```python
from build123d import *

# Parameters (mm, degrees)
SKETCH1_R           = 6
BOSS_EXTRUDE1_DEPTH = 5


with BuildPart() as part:
    # Sketch1 → Boss-Extrude1 (new, symmetric)
    with BuildSketch(Plane.XY):
        with BuildLine():
            ThreePointArc((0, -10), (9.930121511, -1.180121511), (2.34375, 9.721462644))
            Line((2.34375, 9.721462644), (-58.140625, 24.30365661))
            ThreePointArc((-58.140625, 24.30365661), (-86.874486916, 10.08750952), (-77.994140625, -20.716274476))
            ThreePointArc((-77.994140625, -20.716274476), (-72.385268542, -20.708675871), (-70.3125, -15.496849478))
            ThreePointArc((-70.3125, -15.496849478), (-71.576881743, -7.794228634), (-72, 0))
            ThreePointArc((-72, 0), (-64, 8), (-56, 0))
            ThreePointArc((-56, 0), (-55.051774585, -10.261681883), (-52.239210176, -20.175849925))
            ThreePointArc((-52.239210176, -20.175849925), (-46.886715458, -25.748635939), (-39.160382636, -25.843107024))
            Line((-39.160382636, -25.843107024), (0, -10))
        make_face()
        Circle(SKETCH1_R, mode=Mode.SUBTRACT)
    extrude(amount=BOSS_EXTRUDE1_DEPTH, both=True)


solid = part.part
```
Can you work these out from the model? Positions are in its coordinate system, mm. A direction names the side the tool comes from. Coordinates: 2 decimals unless noted, no trailing zeros. Loops run counter-clockwise (first coordinate to the right, second up) from the corner with the lowest first, then second, coordinate; pieces in that order, holes last.
1) Imagine slicing it at D-D on y = 5. List the corners of the cut face in (x, z) for me (3 decimals).
2) I need wall thicknesses on probe 1 along X at (y, z) = (-0.5, 2.25) (1 decimal); probe 2 along Y at (x, z) = (0, 2.25); probe 3 along X at (y, z) = (-14.5, 0). Which ranges of each line are inside material? Lowest first, please.
3) Imagine slicing it at A-A on z = 1. List the corners of the cut face in (x, y) for me, plus the area to 3 significant figures.
4) Imagine slicing it at C-C on x = -64. List the corners of the cut face in (y, z) for me.
5) For pin 1 (11 mm diameter, centred on x = 0, y = 0, fed in from +Z); pin 2 (1.5 mm diameter, centred on x = -67, z = 0, fed in from +Y); pin 3 (1.5 mm diameter, centred on x = -24, z = -1, fed in from -Y); pin 4 (4 mm diameter, centred on y = 10, z = 2.5, fed in from -X), each with a flat end and sliding along its axis, tell me the tip position at first contact or that it passes through.
6) Which directions (+Z, -Z, +X, -X, +Y, -Y) give clear straight access to the entire face, cutting with the end or side of a thin tool? Please do faces 5 (the flat face through (-19.85, -18.03, 0.07)), 6 (the cylindrical face through (-71.565, -7.903, 0.07)).
7) Imagine slicing it at B-B on y = -2. List the corners of the cut face in (x, z) for me.
8) Thinking about a two-plate mould opening in Y: for faces 1 (the cylindrical face through (-64, 8, 0)), 2 (the flat face through (-40, 0, 5)), 3 (the cylindrical face through (9.9, -1.4, 0.1)), 4 (the cylindrical face through (-55.08, -10.12, 0.07)), which applies, pulls with the +Y half, pulls with the -Y half, needs draft (parallel to the pull), parting line crosses it, or undercut?
Completed:
1. outline: (-88.495, -5) - (-70.245, -5) - (-70.245, 5) - (-88.495, 5) - close; (-57.755, -5) - (-3.317, -5) - (-3.317, 5) - (-57.755, 5) - close; (3.317, -5) - (8.66, -5) - (8.66, 5) - (3.317, 5) - close
2. probe 1: x = -89 to -72, -56 to -6, 6 to 10
2. probe 2: y = -10 to -6, 6 to 10.29
2. probe 3: x = -84.37 to -70.52, -54.09 to -11.12
3. outline: (-77.99, -20.72) arc R5 ccw to (-70.31, -15.5) arc R72 cw to (-72, 0) arc R8 cw to (-56, 0) arc R56 ccw to (-52.24, -20.18) arc R10 ccw to (-39.16, -25.84) - (0, -10) arc R10 ccw to (2.34, 9.72) - (-58.14, 24.3) arc R25 ccw to start; hole circle Ø12 at (0, 0)
3. area: 2,970 mm2
4. outline: (8, -5) - (25, -5) - (25, 5) - (8, 5) - close
5. pin 1: passes through
5. pin 2: stops at y = 24.9
5. pin 3: stops at y = -20.01
5. pin 4: stops at x = -87.69
6. face 5: +Z, -Z, +X, -Y
6. face 6: +Z, -Z
7. outline: (-88.92, -5) - (-71.97, -5) - (-71.97, 5) - (-88.92, 5) - close; (-55.96, -5) - (-5.66, -5) - (-5.66, 5) - (-55.96, 5) - close; (5.66, -5) - (9.8, -5) - (9.8, 5) - (5.66, 5) - close
8. face 1: undercut
8. face 2: needs draft
8. face 3: parting line crosses it
8. face 4: pulls with the -Y half
